Design review of the part built by this model. Coordinates are the model's own, in mm. Face numbers are marked on the shaded views. Coordinates: 2 decimals unless noted, no trailing zeros. Order: outer loops, then holes, each group sorted by start corner. A loop starts at its lowest first (then second) coordinate and runs counter-clockwise, first axis right, second up. Notation, with made-up numbers: (-9, 41.5) - (9, 41.5) arc R12 ccw to (9, 53.5) - close; hole circle Ø9 at (31, 3). An arc over 180 degrees is marked (long way). Write item = value, one per line. Start each with the question number.
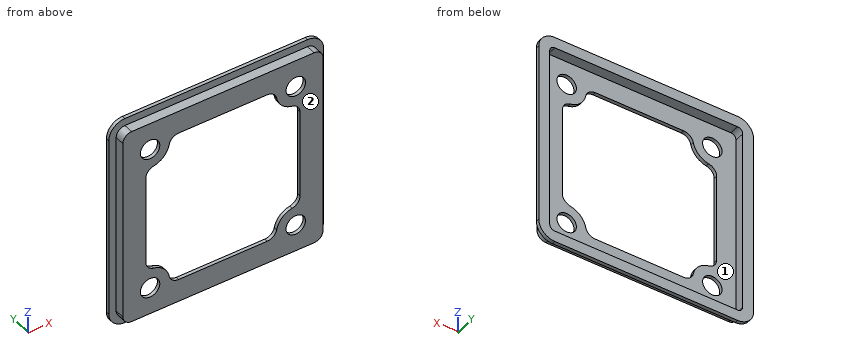
```python
from build123d import *

# Parameters (mm, degrees)
SKETCH1_W           = 103
SKETCH1_H           = 103
SKETCH1_R           = 5
BOSS_EXTRUDE1_DEPTH = 1.8
SKETCH2_W           = 103
SKETCH2_H           = 103
SKETCH2_W_2         = 99.4
SKETCH2_H_2         = 99.4
BOSS_EXTRUDE2_DEPTH = 6.8
FILLET1_R           = 4.5
SKETCH3_W           = 99.4
SKETCH3_H           = 99.4
BOSS_EXTRUDE3_DEPTH = 1.8
FILLET3_R           = 2.7
CUT_EXTRUDE2_DEPTH  = 79.365681264


with BuildPart() as part:
    # Sketch1 → Boss-Extrude1 (new body)
    with BuildSketch(Plane(origin=(0, 0, 0), x_dir=(1, 0, 0), z_dir=(0, 1, 0))):
        Rectangle(SKETCH1_W, SKETCH1_H)
        with Locations(Location((-37.5, 37.5, 0), (0, 0, 270))):
            Circle(SKETCH1_R, mode=Mode.SUBTRACT)
        with Locations(Location((37.5, 37.5, 0), (0, 0, 90))):
            Circle(SKETCH1_R, mode=Mode.SUBTRACT)
        with Locations(Location((37.5, -37.5, 0), (0, 0, 270))):
            Circle(SKETCH1_R, mode=Mode.SUBTRACT)
        with Locations(Location((-37.5, -37.5, 0), (0, 0, 90))):
            Circle(SKETCH1_R, mode=Mode.SUBTRACT)
    extrude(amount=BOSS_EXTRUDE1_DEPTH)

    # Sketch2 → Boss-Extrude2 (add)
    with BuildSketch(Plane.XZ):
        Rectangle(SKETCH2_W, SKETCH2_H)
        Rectangle(SKETCH2_W_2, SKETCH2_H_2, mode=Mode.SUBTRACT)
    extrude(amount=-BOSS_EXTRUDE2_DEPTH)

    # Fillet1
    fillet1_edges = [part.edges().sort_by_distance(p)[0] for p in [
        (51.5, 3.4, 51.5),
        (-51.5, 3.4, 51.5),
        (-51.5, 3.4, -51.5),
        (51.5, 3.4, -51.5),
    ]]
    fillet(fillet1_edges, radius=FILLET1_R)

    # Sketch3 → Boss-Extrude3 (add)
    with BuildSketch(Plane(origin=(0, 6.8, 0), x_dir=(1, 0, 0), z_dir=(0, 1, 0))):
        with BuildLine():
            Line((47, 55.3), (-47, 55.3))
            ThreePointArc((-47, 55.3), (-52.868986284, 52.868986284), (-55.3, 47))
            Line((-55.3, 47), (-55.3, -47))
            ThreePointArc((-55.3, -47), (-52.868986284, -52.868986284), (-47, -55.3))
            Line((-47, -55.3), (47, -55.3))
            ThreePointArc((47, -55.3), (52.868986284, -52.868986284), (55.3, -47))
            Line((55.3, -47), (55.3, 47))
            ThreePointArc((55.3, 47), (52.868986284, 52.868986284), (47, 55.3))
        make_face()
        Rectangle(SKETCH3_W, SKETCH3_H, mode=Mode.SUBTRACT)
    extrude(amount=-BOSS_EXTRUDE3_DEPTH)

    # Fillet3
    fillet3_edges = [part.edges().sort_by_distance(p)[0] for p in [
        (-49.7, 4.3, 49.7),
        (-49.7, 4.3, -49.7),
        (49.7, 4.3, -49.7),
        (49.7, 4.3, 49.7),
    ]]
    fillet(fillet3_edges, radius=FILLET3_R)

    # Sketch5 → Cut-Extrude2 (cut, through all)
    with BuildSketch(Plane(origin=(0, 1.8, 0), x_dir=(1, 0, 0), z_dir=(0, 1, 0))):
        with BuildLine():
            Line((22.763650384, 39.7), (-22.763650384, 39.7))
            ThreePointArc((-22.763650384, 39.7), (-25.952171462, 38.551406669), (-27.675766923, 35.633333333))
            ThreePointArc((-27.675766923, 35.633333333), (-30.428932188, 30.428932188), (-35.633333333, 27.675766923))
            ThreePointArc((-35.633333333, 27.675766923), (-38.551406669, 25.952171462), (-39.7, 22.763650384))
            Line((-39.7, 22.763650384), (-39.7, -22.763650384))
            ThreePointArc((-39.7, -22.763650384), (-38.551406669, -25.952171462), (-35.633333333, -27.675766923))
            ThreePointArc((-35.633333333, -27.675766923), (-30.428932188, -30.428932188), (-27.675766923, -35.633333333))
            ThreePointArc((-27.675766923, -35.633333333), (-25.952171462, -38.551406669), (-22.763650384, -39.7))
            Line((-22.763650384, -39.7), (22.763650384, -39.7))
            ThreePointArc((22.763650384, -39.7), (25.952171462, -38.551406669), (27.675766923, -35.633333333))
            ThreePointArc((27.675766923, -35.633333333), (30.428932188, -30.428932188), (35.633333333, -27.675766923))
            ThreePointArc((35.633333333, -27.675766923), (38.551406669, -25.952171462), (39.7, -22.763650384))
            Line((39.7, -22.763650384), (39.7, 22.763650384))
            ThreePointArc((39.7, 22.763650384), (38.551406669, 25.952171462), (35.633333333, 27.675766923))
            ThreePointArc((35.633333333, 27.675766923), (30.428932188, 30.428932188), (27.675766923, 35.633333333))
            ThreePointArc((27.675766923, 35.633333333), (25.952171462, 38.551406669), (22.763650384, 39.7))
        make_face()
    extrude(amount=-CUT_EXTRUDE2_DEPTH, mode=Mode.SUBTRACT)


solid = part.part
```
Item 1: Mouldability with a two-part tool opening along X and no side actions: class the marked faces 1 and 2 as +X half, -X half, draft (parallel to the pull), parting line (faces both ways), or undercut.
Item 2: For line 1 (Z direction, x = 7, y = 1); line 2 (X direction, y = 2.25, z = -21.5); line 3 (X direction, y = 1.1, z = 37.5), list the stretches that pass through material, from the lowest coordinate up.
Item 3: Add section B-B on y = 3. Give the boundary of the cut face in (x, z).
Item 4: Add section D-D on z = -34. Give the boundary of the cut face in (x, y), plus the area to 3 significant figures.
Item 5: Add section A-A on z = -11. Give the boundary of the cut face in (x, y), plus the area to 3 significant figures.
Item 6: For P1, Ø1.5, axis at y = 4, z = 9.5, coming from the -X side; P2, Ø1, axis at x = -39.5, y = 2.5, coming from the -Z side; P3, Ø2.5, axis at x = -12, y = 1.5, coming from the +Z side, all flat-tipped, find the tip position at first contact; note any pin that passes through.
Item 7: Add section C-C on x = 5. Give the boundary of the cut face in (y, z), plus the area to 3 significant figures.
Worked out:
q1.face_1 = undercut
q1.face_2 = draft
q2.line_1 = -51.5 to -39.7, 39.7 to 51.5
q2.line_2 = -51.5 to -49.7, 49.7 to 51.5
q2.line_3 = -51.5 to -42.5, -32.5 to -26.91, 26.91 to 32.5, 42.5 to 51.5
q3.outline = (-51.5, -47) arc R4.5 ccw to (-47, -51.5) - (47, -51.5) arc R4.5 ccw to (51.5, -47) - (51.5, 47) arc R4.5 ccw to (47, 51.5) - (-47, 51.5) arc R4.5 ccw to (-51.5, 47) - close; hole (-49.7, -47) arc R2.7 ccw to (-47, -49.7) - (47, -49.7) arc R2.7 ccw to (49.7, -47) - (49.7, 47) arc R2.7 ccw to (47, 49.7) - (-47, 49.7) arc R2.7 ccw to (-49.7, 47) - close
q4.outline = (-55.3, 5) - (-51.5, 5) - (-51.5, 0) - (-41.07, 0) - (-41.07, 1.8) - (-49.7, 1.8) - (-49.7, 6.8) - (-55.3, 6.8) - close; (-33.93, 0) - (-28.13, 0) - (-28.13, 1.8) - (-33.93, 1.8) - close; (28.13, 0) - (33.93, 0) - (33.93, 1.8) - (28.13, 1.8) - close; (41.07, 0) - (51.5, 0) - (51.5, 5) - (55.3, 5) - (55.3, 6.8) - (49.7, 6.8) - (49.7, 1.8) - (41.07, 1.8) - close
q4.area = 90.1 mm2
q5.outline = (-55.3, 5) - (-51.5, 5) - (-51.5, 0) - (-39.7, 0) - (-39.7, 1.8) - (-49.7, 1.8) - (-49.7, 6.8) - (-55.3, 6.8) - close; (39.7, 0) - (51.5, 0) - (51.5, 5) - (55.3, 5) - (55.3, 6.8) - (49.7, 6.8) - (49.7, 1.8) - (39.7, 1.8) - close
q5.area = 74.2 mm2
q6.P1 = -51.5
q6.P2 = -51.5
q6.P3 = 51.5
q7.outline = (0, -51.5) - (5, -51.5) - (5, -55.3) - (6.8, -55.3) - (6.8, -49.7) - (1.8, -49.7) - (1.8, -39.7) - (0, -39.7) - close; (0, 39.7) - (1.8, 39.7) - (1.8, 49.7) - (6.8, 49.7) - (6.8, 55.3) - (5, 55.3) - (5, 51.5) - (0, 51.5) - close
q7.area = 74.2 mm2
